Read the model definition and answer for the solid it produces. Units are mm, in the model's axes. Give positions to 0.01 mm unless a question says otherwise; leave off trailing zeros. Write each loop counter-clockwise with the first axis right and the second up, starting at its lowest first coordinate (ties: lowest second). Pieces come first, ordered by that corner, then holes. Notation, with made-up numbers: M 10,84.5 L 49,84.5 A25 ccw 49,103.5 Z; hole C 10.25,25 d1. An arc over 180 degrees is marked long. Put each result on its own line as item: value.
from build123d import *

# Parameters (mm, degrees)
F1_DEPTH = 7.5
F2_R     = 2
F3_SIZE  = 1


with BuildPart() as f1:
    # F0 (on Front) → F1 (new body)
    with BuildSketch(Plane.XZ):
        with BuildLine():
            Line((7.648719, 8.582773), (-8.586255, 8.582773))
            Line((-8.586255, 8.582773), (-8.586255, 5.043917))
            Line((-8.586255, 5.043917), (0.670703, 5.043917))
            ThreePointArc((0.670703, 5.043917), (8.022373, -0.80316), (7.648719, 8.582773))
        make_face()
    extrude(amount=F1_DEPTH)

    # F2
    f2_edges = [f1.edges().sort_by_distance(p)[0] for p in [
        (-8.586255, -3.75, 5.043917),
    ]]
    fillet(f2_edges, radius=F2_R)

    # F3
    f3_edges = [f1.edges().sort_by_distance(p)[0] for p in [
        (-8.586255, -3.75, 8.582773),
    ]]
    chamfer(f3_edges, length=F3_SIZE)


solid = f1.part
(1) Section A-A on y = -5.25 is taken. Determine the outline of the cut face in (x, z), and give its area (3 significant figures).
Result:
outline: M -8.59,7.04 A2 ccw -6.59,5.04 L 0.67,5.04 A5.17 ccw long 7.65,8.58 L -7.59,8.58 L -8.59,7.58 Z
area: 118 mm²
(2) Given pin 1 Ø1 at (y, z) = (-2, 5) entering from -X, flat-ended and moving along its own axis, determine where the tip first touches the part or whether it passes through.
Result:
pin 1: stops at x = -7.86
(3) Section C-C on z = 2.25 is taken. Determine the outline of the cut face in (x, y).
Result:
outline: M 0.76,-7.5 L 10.61,-7.5 L 10.61,0 L 0.76,0 Z
(4) Straight lines are drawn through the part: line 1 along Z through (x, y) = (-3.5, -1.5); line 2 along Z through (x, y) = (-7.75, -0.25); line 3 along X through (y, z) = (-3, 6.25). For each, find the intervals that lie inside material, in ascending order. Write a range as from..to.
Result:
line 1: z = 5.04..8.58
line 2: z = 5.42..8.42
line 3: x = -8.42..10.24
(5) Section B-B on x = -0.5 is taken. Determine the outline of the cut face in (y, z), and give its area (3 significant figures).
Result:
outline: M -7.5,5.04 L 0,5.04 L 0,8.58 L -7.5,8.58 Z
area: 26.5 mm²
